```python
from build123d import *

# Parameters (mm, degrees)
F0_W     = 45
F0_H     = 22
F1_DEPTH = 1.6
F2_W     = 45
F2_H     = 1.6
F3_DEPTH = 25
F4_R     = 2
F5_DEPTH = 25
F6_R     = 2


with BuildPart() as f1:
    # F0 (on Right) → F1 (new body)
    with BuildSketch(Plane.YZ):
        with Locations((3.901578, -0.626537)):
            Rectangle(F0_W, F0_H)
    extrude(amount=F1_DEPTH)

    # F2 (on face) → F3 (join)
    with BuildSketch(Plane(origin=(0, 0, 0), x_dir=(0, -1, 0), z_dir=(-1, 0, 0))):
        with Locations((-3.901578, 9.573463)):
            Rectangle(F2_W, F2_H)
        with Locations((-3.901578, -10.826537)):
            Rectangle(F2_W, F2_H)
    extrude(amount=F3_DEPTH)

    # F4 (on face) → F5 (cut)
    with BuildSketch(Plane.XY.offset(10.373463)):
        with BuildLine():
            Line((-25, -18.598422), (-4.034702, -18.598422))
            ThreePointArc((-4.034702, -18.598422), (-5.277364, -18.328951), (-6.296786, -17.568949))
            Line((-6.296786, -17.568949), (-23.283452, 1.931051))
            ThreePointArc((-23.283452, 1.931051), (-24.021368, 3.901578), (-23.283452, 5.872105))
            Line((-23.283452, 5.872105), (-6.296786, 25.372105))
            ThreePointArc((-6.296786, 25.372105), (-5.277364, 26.132107), (-4.034702, 26.401578))
            Line((-4.034702, 26.401578), (-25, 26.401578))
            Line((-25, 26.401578), (-25, -18.598422))
        make_face()
        with Locations((-21.021368, 3.901578)):
            Circle(F4_R)
    extrude(amount=-F5_DEPTH, mode=Mode.SUBTRACT)

    # F6
    f6_edges = [f1.edges().sort_by_distance(p)[0] for p in [
        (1.6, 3.901578, -11.626537),
        (1.6, 3.901578, 10.373463),
        (0, 3.901578, -10.026537),
        (0, 3.901578, 8.773463),
    ]]
    fillet(f6_edges, radius=F6_R)


solid = f1.part
```
For this review, take the finished solid that the model builds, in its own axes (mm). A direction names the side the tool comes from. Round coordinates to 2 decimals unless told otherwise and drop trailing zeros. Write each loop counter-clockwise with the first axis right and the second up, starting at its lowest first coordinate (ties: lowest second). Pieces come first, ordered by that corner, then holes. Notation, with made-up numbers: (85.5, -40) - (129.5, -40) arc R19 cw to (129.5, -21) - close; hole circle Ø4 at (65, 84). An arc over 180 degrees is marked (long way). Put each result on its own line as item: value.
Q1. We need section C-C (y = 5). Give the boundary of the cut face in (x, z), and give its area (3 significant figures).
Solved:
outline: (-23.81, -11.63) - (-22.69, -11.63) - (-22.69, -10.03) - (-23.81, -10.03) - close; (-23.81, 8.77) - (-22.69, 8.77) - (-22.69, 10.37) - (-23.81, 10.37) - close; (-19.35, -11.63) - (-0.4, -11.63) arc R2 ccw to (1.6, -9.63) - (1.6, 8.37) arc R2 ccw to (-0.4, 10.37) - (-19.35, 10.37) - (-19.35, 8.77) - (-2, 8.77) arc R2 cw to (0, 6.77) - (0, -8.03) arc R2 cw to (-2, -10.03) - (-19.35, -10.03) - close
area: 101 mm2
Q2. Wall thickness on probe 1 along Z at (x, y) = (-8.25, 19); probe 2 along X at (y, z) = (22.5, 4.75); probe 3 along Z at (x, y) = (-1, 4): over which ranges is each line inside the solid? List them lowest first.
Solved:
probe 1: z = -11.63 to -10.03, 8.77 to 10.37
probe 2: x = 0 to 1.6
probe 3: z = -11.63 to -9.76, 8.51 to 10.37
Q3. Machinability: for faces 1 (the face through (-14.909, 15.486, -10.815)), 2 (the face through (-0.57, 3.587, -9.425)), which of the approach directions +Z, -Z, +X, -X, +Y, -Y give a long, thin tool a straight path to every point of the face, cutting with its end or side? Answer none if there is none.
Solved:
face 1: +Z, -Z, -X, +Y
face 2: -X, +Y, -Y
Q4. We need section B-B (x = -16). Give the boundary of the cut face in (y, z), and give its area (3 significant figures).
Solved:
outline: (-6.43, -11.63) - (14.23, -11.63) - (14.23, -10.03) - (-6.43, -10.03) - close; (-6.43, 8.77) - (14.23, 8.77) - (14.23, 10.37) - (-6.43, 10.37) - close
area: 66.1 mm2
Q5. We need section A-A (x = -20.5). Give the boundary of the cut face in (y, z).
Solved:
outline: (-1.26, -11.63) - (1.97, -11.63) - (1.97, -10.03) - (-1.26, -10.03) - close; (-1.26, 8.77) - (1.97, 8.77) - (1.97, 10.37) - (-1.26, 10.37) - close; (5.83, -11.63) - (9.07, -11.63) - (9.07, -10.03) - (5.83, -10.03) - close; (5.83, 8.77) - (9.07, 8.77) - (9.07, 10.37) - (5.83, 10.37) - close
Q6. Insertion check: pin 1 Ø8 at (x, y) = (-19.5, -7.5) entering from +Z; pin 2 Ø2 at (y, z) = (-13, 5) entering from -X. Each pin has a flat end and moves straight along its axis. Give the tip position at first contact, or say it passes through.
Solved:
pin 1: stops at z = 10.37
pin 2: stops at x = 0
Q7. We need section D-D (z = -3). Give the boundary of the cut face in (x, y).
Solved:
outline: (0, -18.6) - (1.6, -18.6) - (1.6, 26.4) - (0, 26.4) - close
Q8. Mouldability with a two-part tool opening along Z and no side actions: class faces 3 (the face through (-14.671, -7.955, 9.585)), 4 (the face through (0, 4, -1)), 5 (the face through (0.999, 4.217, -11.056)) as released by +Z, released by -Z, zero draft, split by the parting line, or undercut.
Solved:
face 3: zero draft
face 4: undercut
face 5: released by -Z
